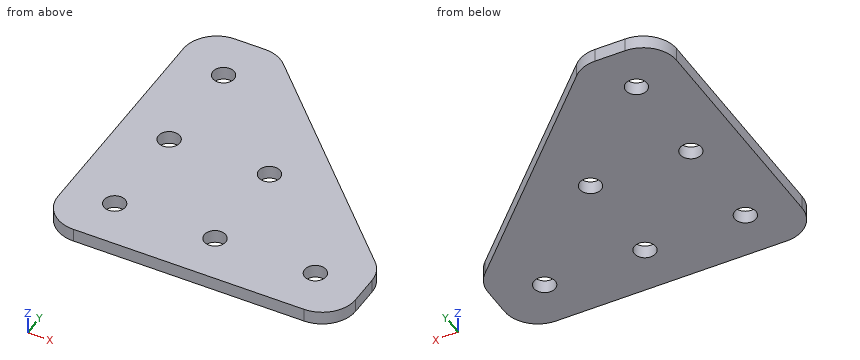
```python
from build123d import *

# Parameters (mm, degrees)
SKETCH1_R           = 1.6
BOSS_EXTRUDE1_DEPTH = 2


with BuildPart() as part:
    # Sketch1 → Boss-Extrude1 (new body)
    with BuildSketch(Plane.XY):
        with BuildLine():
            Line((13.035533906, 43.035533906), (43.035533906, 13.035533906))
            ThreePointArc((43.035533906, 13.035533906), (44.119397663, 11.413417162), (44.5, 9.5))
            Line((44.5, 9.5), (44.5, 5))
            ThreePointArc((44.5, 5), (43.035533906, 1.464466094), (39.5, 0))
            Line((39.5, 0), (5, 0))
            ThreePointArc((5, 0), (1.464466094, 1.464466094), (0, 5))
            Line((0, 5), (0, 39.5))
            ThreePointArc((0, 39.5), (1.464466094, 43.035533906), (5, 44.5))
            Line((5, 44.5), (9.5, 44.5))
            ThreePointArc((9.5, 44.5), (11.413417162, 44.119397663), (13.035533906, 43.035533906))
        make_face()
        with Locations((7.25, 7.25)):
            Circle(SKETCH1_R, mode=Mode.SUBTRACT)
        with Locations((7.25, 22.25)):
            Circle(SKETCH1_R, mode=Mode.SUBTRACT)
        with Locations((7.25, 37.25)):
            Circle(SKETCH1_R, mode=Mode.SUBTRACT)
        with Locations((22.25, 7.25)):
            Circle(SKETCH1_R, mode=Mode.SUBTRACT)
        with Locations((37.25, 7.25)):
            Circle(SKETCH1_R, mode=Mode.SUBTRACT)
        with Locations((22.25, 22.25)):
            Circle(SKETCH1_R, mode=Mode.SUBTRACT)
    extrude(amount=BOSS_EXTRUDE1_DEPTH)


solid = part.part
```
Can you work these out from the model? Positions are in its coordinate system, mm. Coordinates: 2 decimals unless noted, no trailing zeros. Write each loop counter-clockwise with the first axis right and the second up, starting at its lowest first coordinate (ties: lowest second). Pieces come first, ordered by that corner, then holes. Notation, with made-up numbers: M -28,32.25 L -12,32.25 A21 ccw -12,60.25 Z; hole C 86,26.5 d6. An arc over 180 degrees is marked long. Write item = value, one per line. Start each with the question number.
Q1. If we section it at A-A, the plane z = 1.25: Write out the boundary of the cut face in (x, y), then the cut area to 3 significant figures.
Q2. If we section it at D-D, the plane y = 22.25: Write out the boundary of the cut face in (x, z).
Q3. If we section it at B-B, the plane x = 7.25: Write out the boundary of the cut face in (y, z).
Q4. If I drill on L1, parallel to Y at x = 7.25, z = 0.55; L2, parallel to X at y = 22, z = 1.7; L3, parallel to Y at x = 22.25, z = 0.65, over which ranges is the centre line in solid material (lowest first)? Write a range as [from, to].
Check sheet entries:
q1.outline = M 0,5 A5 ccw 5,0 L 39.5,0 A5 ccw 44.5,5 L 44.5,9.5 A5 ccw 43.04,13.04 L 13.04,43.04 A5 ccw 9.5,44.5 L 5,44.5 A5 ccw 0,39.5 Z; hole C 7.25,7.25 d3.2; hole C 7.25,22.25 d3.2; hole C 7.25,37.25 d3.2; hole C 22.25,7.25 d3.2; hole C 22.25,22.25 d3.2; hole C 37.25,7.25 d3.2
q1.area = 1,370 mm²
q2.outline = M 0,0 L 5.65,0 L 5.65,2 L 0,2 Z; M 8.85,0 L 20.65,0 L 20.65,2 L 8.85,2 Z; M 23.85,0 L 33.82,0 L 33.82,2 L 23.85,2 Z
q3.outline = M 0,0 L 5.65,0 L 5.65,2 L 0,2 Z; M 8.85,0 L 20.65,0 L 20.65,2 L 8.85,2 Z; M 23.85,0 L 35.65,0 L 35.65,2 L 23.85,2 Z; M 38.85,0 L 44.5,0 L 44.5,2 L 38.85,2 Z
q4.L1 = [0, 5.65], [8.85, 20.65], [23.85, 35.65], [38.85, 44.5]
q4.L2 = [0, 5.67], [8.83, 20.67], [23.83, 34.07]
q4.L3 = [0, 5.65], [8.85, 20.65], [23.85, 33.82]
